from build123d import *

# Parameters (mm, degrees)
BOSS_EXTRUDE1_DEPTH = 1518.68
SHELL1_T            = -6.35
CUT_EXTRUDE2_REACH  = 1775.764
SKETCH3_W           = 277
SKETCH3_H           = 50


with BuildPart() as part:
    # Sketch1 → Boss-Extrude1 (new body)
    with BuildSketch(Plane(origin=(0, 0, 0), x_dir=(0, 0, -1), z_dir=(1, 0, 0))):
        Polygon((0, 403.229130413), (0, 0), (829.306608812, 0), (829.306608812, 257), align=None)
    extrude(amount=BOSS_EXTRUDE1_DEPTH)

    # Shell1
    shell1_openings = [part.faces().sort_by_distance(p)[0] for p in [
        (759.34, 330.114565207, -414.653304406),
        (759.34, 0, -414.653304406),
    ]]
    offset(amount=SHELL1_T, openings=shell1_openings, kind=Kind.INTERSECTION)

    # Sketch3 → Cut-Extrude2 (cut, up to next)
    with BuildSketch(Plane.XY.offset(-822.956608812), mode=Mode.PRIVATE) as cut_extrude2_sk1:
        with Locations((462.5, 243.119676327)):
            Rectangle(SKETCH3_W, SKETCH3_H)
    cut_extrude2_tool1 = extrude(cut_extrude2_sk1.sketch, amount=-CUT_EXTRUDE2_REACH, mode=Mode.PRIVATE) & part.part
    add(cut_extrude2_tool1.solids().sort_by_distance((462.5, 243.119676, -822.956609))[0], mode=Mode.SUBTRACT)


solid = part.part
Geometry check sheet. Reference: the model listing, model coordinates, mm. A direction names the side the tool comes from. Round coordinates to 2 decimals unless told otherwise and drop trailing zeros. Loops run counter-clockwise (first coordinate to the right, second up) from the corner with the lowest first, then second, coordinate; pieces in that order, holes last.
Item 1: Gauge pin test, flat end, axial feed: pin 1 (5 mm diameter, centred on x = 453.5, z = -825.5, fed in from +Y). Record the tip position at first contact, or that the pin passes through.
Item 2: Cross-section at D-D on y = 360. Record the boundary of the cut face in (x, z), then the cut area to 3 significant figures.
Item 3: Access from +Z, -Z, +X, -X, +Y, -Y to the whole of each face (thin tool, end or side, straight path). Record for faces 4 (the flat face through (749, 204, -6.35)), 5 (the flat face through (749, 127, -829.307)).
Item 4: Cross-section at C-C on y = 169.5. Record the boundary of the cut face in (x, z).
Item 5: Cross-section at B-B on z = -388.5. Record the boundary of the cut face in (x, y).
Item 6: Thickness scan on line 1 (X direction, y = 99, z = -142); line 2 (Z direction, x = 418.5, y = 124.5); line 3 (Z direction, x = 787, y = 366.5). Record the ranges inside material, lowest first.
Item 7: Cross-section at A-A on x = 564. Record the boundary of the cut face in (y, z), then the cut area to 3 significant figures.
Item 8: Mould release check, pull along Z, two halves, no side actions. Record for faces 1 (the flat face through (749, 204, 0)), 2 (the flat face through (1518.68, 160, -409)), 3 (the flat face through (1512.33, 159, -409)): pulls with the +Z half, pulls with the -Z half, needs draft (parallel to the pull), parting line crosses it, or undercut.
Answer sheet:
1. pin 1: stops at y = 218.12
2. outline: (0, -245.16) - (6.35, -245.16) - (6.35, -6.35) - (1512.33, -6.35) - (1512.33, -245.16) - (1518.68, -245.16) - (1518.68, 0) - (0, 0) - close
2. area: 12,700 mm2
3. face 4: +Y, -Y
3. face 5: -Z, +X, -X, +Y, -Y
4. outline: (0, -829.31) - (1518.68, -829.31) - (1518.68, 0) - (0, 0) - close; hole (6.35, -822.96) - (1512.33, -822.96) - (1512.33, -6.35) - (6.35, -6.35) - close
5. outline: (0, 0) - (6.35, 0) - (6.35, 334.73) - (0, 334.73) - close; (1512.33, 0) - (1518.68, 0) - (1518.68, 334.73) - (1512.33, 334.73) - close
6. line 1: x = 0 to 6.35, 1512.33 to 1518.68
6. line 2: z = -829.31 to -822.96, -6.35 to 0
6. line 3: z = -6.35 to 0
7. outline: (0, -829.31) - (218.12, -829.31) - (218.12, -822.96) - (0, -822.96) - close; (0, -6.35) - (402.11, -6.35) - (403.23, 0) - (0, 0) - close
7. area: 3,940 mm2
8. face 1: pulls with the +Z half
8. face 2: needs draft
8. face 3: undercut
